```python
from build123d import *

# Parameters (mm, degrees)
UPPER_BOARD_R   = 9
UPPER_BOARD_R_2 = 1.75
UPPER_BOARD_R_3 = 1.65
EXTRUDE_1_DEPTH = 1.5


with BuildPart() as part:
    # Upper_board → 凸台-拉伸1 (new body)
    with BuildSketch(Plane.XY):
        Polygon((0, 29.63770528), (9.258229776, 29.63770528), (13.530145247, 31.914413679), (21.845237215, 38.947274579), (39.422116781, 21.483203913), (39.422116781, 17.759375685), (45.602672711, 13.431703833), (47.117107925, 11.564161962), (47.117107925, -11.564161962), (45.602672711, -13.431703833), (39.422116781, -17.759375685), (39.422116781, -21.483203913), (21.845237215, -38.947274579), (13.530145247, -31.914413679), (9.258229776, -29.63770528), (0, -29.63770528), (-8.800437365, -29.63770528), (-11.64882797, -31.155749084), (-21.754927214, -39.351031245), (-38.850540354, -22.144989251), (-38.878084859, -15.364158174), (-43.219581062, -15.364158174), (-44.585312397, -13.989604918), (-44.585312397, 13.989604918), (-43.219581062, 15.364158174), (-38.878084859, 15.364158174), (-38.850540354, 22.144989251), (-21.754927214, 39.351031245), (-11.64882797, 31.155749084), (-8.800437365, 29.63770528), align=None)
        Circle(UPPER_BOARD_R, mode=Mode.SUBTRACT)
        with Locations((-20.893398282, 31.606601718)):
            Circle(UPPER_BOARD_R_2, mode=Mode.SUBTRACT)
        with Locations((-31.5, 21)):
            Circle(UPPER_BOARD_R_2, mode=Mode.SUBTRACT)
        with Locations((-33.5, 0)):
            Circle(UPPER_BOARD_R_3, mode=Mode.SUBTRACT)
        with Locations(Location((20.893398282, 31.606601718, 0), (0, 0, 180))):
            Circle(UPPER_BOARD_R_2, mode=Mode.SUBTRACT)
        with Locations(Location((31.5, 21, 0), (0, 0, 180))):
            Circle(UPPER_BOARD_R_2, mode=Mode.SUBTRACT)
        with Locations(Location((-20.893398282, -31.606601718, 0), (0, 0, 180))):
            Circle(UPPER_BOARD_R_2, mode=Mode.SUBTRACT)
        with Locations(Location((-31.5, -21, 0), (0, 0, 180))):
            Circle(UPPER_BOARD_R_2, mode=Mode.SUBTRACT)
        with Locations((20.893398282, -31.606601718)):
            Circle(UPPER_BOARD_R_2, mode=Mode.SUBTRACT)
        with Locations((31.5, -21)):
            Circle(UPPER_BOARD_R_2, mode=Mode.SUBTRACT)
        with BuildLine():
            Line((-21.566327477, 23.687647821), (-10.960584458, 13.081904801))
            ThreePointArc((-10.960584458, 13.081904801), (-10.960584458, 10.960584458), (-13.081904801, 10.960584458))
            Line((-13.081904801, 10.960584458), (-23.687647821, 21.566327477))
            ThreePointArc((-23.687647821, 21.566327477), (-23.687647821, 23.687647821), (-21.566327477, 23.687647821))
        make_face(mode=Mode.SUBTRACT)
        with BuildLine():
            Line((-1.5, 17.445654013), (-1.5, 25.945654013))
            ThreePointArc((-1.5, 25.945654013), (0, 27.445654013), (1.5, 25.945654013))
            Line((1.5, 25.945654013), (1.5, 17.445654013))
            ThreePointArc((1.5, 17.445654013), (0, 15.945654013), (-1.5, 17.445654013))
        make_face(mode=Mode.SUBTRACT)
        with BuildLine():
            Line((-1.5, -17.445654013), (-1.5, -25.945654013))
            ThreePointArc((-1.5, -25.945654013), (0, -27.445654013), (1.5, -25.945654013))
            Line((1.5, -25.945654013), (1.5, -17.445654013))
            ThreePointArc((1.5, -17.445654013), (0, -15.945654013), (-1.5, -17.445654013))
        make_face(mode=Mode.SUBTRACT)
        with BuildLine():
            Line((-17.445654013, 1.5), (-25.945654013, 1.5))
            ThreePointArc((-25.945654013, 1.5), (-27.445654013, 0), (-25.945654013, -1.5))
            Line((-25.945654013, -1.5), (-17.445654013, -1.5))
            ThreePointArc((-17.445654013, -1.5), (-15.945654013, 0), (-17.445654013, 1.5))
        make_face(mode=Mode.SUBTRACT)
        with BuildLine():
            Line((17.445654013, 1.5), (25.945654013, 1.5))
            ThreePointArc((25.945654013, 1.5), (27.445654013, 0), (25.945654013, -1.5))
            Line((25.945654013, -1.5), (17.445654013, -1.5))
            ThreePointArc((17.445654013, -1.5), (15.945654013, 0), (17.445654013, 1.5))
        make_face(mode=Mode.SUBTRACT)
        with BuildLine():
            Line((-21.566327477, -23.687647821), (-10.960584458, -13.081904801))
            ThreePointArc((-10.960584458, -13.081904801), (-10.960584458, -10.960584458), (-13.081904801, -10.960584458))
            Line((-13.081904801, -10.960584458), (-23.687647821, -21.566327477))
            ThreePointArc((-23.687647821, -21.566327477), (-23.687647821, -23.687647821), (-21.566327477, -23.687647821))
        make_face(mode=Mode.SUBTRACT)
        with BuildLine():
            Line((21.566327477, 23.687647821), (10.960584458, 13.081904801))
            ThreePointArc((10.960584458, 13.081904801), (10.960584458, 10.960584458), (13.081904801, 10.960584458))
            Line((13.081904801, 10.960584458), (23.687647821, 21.566327477))
            ThreePointArc((23.687647821, 21.566327477), (23.687647821, 23.687647821), (21.566327477, 23.687647821))
        make_face(mode=Mode.SUBTRACT)
        with BuildLine():
            Line((21.566327477, -23.687647821), (10.960584458, -13.081904801))
            ThreePointArc((10.960584458, -13.081904801), (10.960584458, -10.960584458), (13.081904801, -10.960584458))
            Line((13.081904801, -10.960584458), (23.687647821, -21.566327477))
            ThreePointArc((23.687647821, -21.566327477), (23.687647821, -23.687647821), (21.566327477, -23.687647821))
        make_face(mode=Mode.SUBTRACT)
        with BuildLine():
            Line((-41, -11), (-41, 11))
            ThreePointArc((-41, 11), (-40, 12), (-39, 11))
            Line((-39, 11), (-39, -11))
            ThreePointArc((-39, -11), (-40, -12), (-41, -11))
        make_face(mode=Mode.SUBTRACT)
        with BuildLine():
            Line((41.855351652, -4.5), (41.855351652, 4.5))
            ThreePointArc((41.855351652, 4.5), (42.721395453, 5.366043802), (43.587439255, 4.5))
            Line((43.587439255, 4.5), (43.587439255, -4.5))
            ThreePointArc((43.587439255, -4.5), (42.721395453, -5.366043802), (41.855351652, -4.5))
        make_face(mode=Mode.SUBTRACT)
    extrude(amount=EXTRUDE_1_DEPTH)


solid = part.part
```
Could you check a few things on this model? Use its own coordinates, in mm. A direction names the side the tool comes from. Give positions to 0.01 mm unless a question says otherwise; leave off trailing zeros. Order: outer loops, then holes, each group sorted by start corner. A loop starts at its lowest first (then second) coordinate and runs counter-clockwise, first axis right, second up.
Q1. Suppose I cut it at D-D, the plane z = 1.15. Count the separate pieces of the cut face and the enclosed holes in it, and give its area (3 significant figures).
Q2. If I drill on line 1 along Y through (x, z) = (-31.5, 0.85); line 2 along Y through (x, z) = (-1, 0.9); line 3 along X through (y, z) = (-13.5, 0.25), over which ranges is the centre line in solid material (lowest first)?
Q3. Suppose I cut it at A-A, the plane y = 0. Write out the boundary of the cut face in (x, z).
Q4. For faces 1 (the flat face through (11.36, 30.76, 0.74)), 2 (the flat face through (18.31, -16.19, 0.74)), 3 (the flat face through (11.42, -30.79, 0.74)), which set-ups out of +Z, -Z, +X, -X, +Y, -Y let a thin tool reach every point of the face, with its end or its side?
Q5. Suppose I cut it at B-B, the plane x = -40. Write out the boundary of the cut face in (y, z).
Q6. Suppose I cut it at C-C, the plane x = -3.5. Write out the boundary of the cut face in (y, z), and give its area (3 significant figures).
Q7. We'd pull the mould along Y, two halves only. Please class faces 4 (the flat face through (30.76, -30.09, 0.74)), 5 (the cylindrical face through (-10.94, 10.98, 0.74)), 6 (the flat face through (42.469, 15.626, 0.74)): +Y half, -Y half, draft (parallel to the pull), parting line (faces both ways), or undercut.
Q8. I'm going to push flat-ended pins straight in: P1, Ø0.8, axis at x = 23.5, z = 0.5, coming from the -Y side; P2, Ø0.8, axis at x = -3, z = 0.5, coming from the -Y side; P3, Ø0.8, axis at x = 20.5, z = 0.5, coming from the +Y side. Where does each tip first touch, or does it pass through?
Solution:
1. separate pieces: 1
1. enclosed holes: 20
1. area: 4,580 mm2
2. line 1: y = -29.54 to -22.75, -19.25 to 19.25, 22.75 to 29.54
2. line 2: y = -29.64 to -27.06, -16.33 to -8.94, 8.94 to 16.33, 27.06 to 29.64
2. line 3: x = -44.59 to -15.62, -11.38 to 11.38, 15.62 to 45.51
3. outline: (-44.59, 0) - (-41, 0) - (-41, 1.5) - (-44.59, 1.5) - close; (-39, 0) - (-35.15, 0) - (-35.15, 1.5) - (-39, 1.5) - close; (-31.85, 0) - (-27.45, 0) - (-27.45, 1.5) - (-31.85, 1.5) - close; (-15.95, 0) - (-9, 0) - (-9, 1.5) - (-15.95, 1.5) - close; (9, 0) - (15.95, 0) - (15.95, 1.5) - (9, 1.5) - close; (27.45, 0) - (41.86, 0) - (41.86, 1.5) - (27.45, 1.5) - close; (43.59, 0) - (47.12, 0) - (47.12, 1.5) - (43.59, 1.5) - close
4. face 1: +Z, -Z, +Y
4. face 2: +Z, -Z
4. face 3: +Z, -Z, -Y
5. outline: (-15.36, 0) - (-12, 0) - (-12, 1.5) - (-15.36, 1.5) - close; (12, 0) - (15.36, 0) - (15.36, 1.5) - (12, 1.5) - close
6. outline: (-29.64, 0) - (-8.29, 0) - (-8.29, 1.5) - (-29.64, 1.5) - close; (8.29, 0) - (29.64, 0) - (29.64, 1.5) - (8.29, 1.5) - close
6. area: 64.0 mm2
7. face 4: -Y half
7. face 5: undercut
7. face 6: +Y half
8. P1: stops at y = -37.7
8. P2: stops at y = -29.64
8. P3: stops at y = 38.15
